Source: three-view drawing plus pictorial views. Frame: mm from the lowest corner of the part. A direction names the side the tool comes from. Give positions to 0.01 mm unless a question says otherwise; leave off trailing zeros. Loops run counter-clockwise (first coordinate to the right, second up) from the corner with the lowest first, then second, coordinate; pieces in that order, holes last. Notation, with made-up numbers: M -30.75,-24 L -26.75,-24 A20 cw -26.75,-19 Z; hole C 89.25,22 d2. An arc over 180 degrees is marked long. Put each result on its own line as item: value. Start each with the question number.
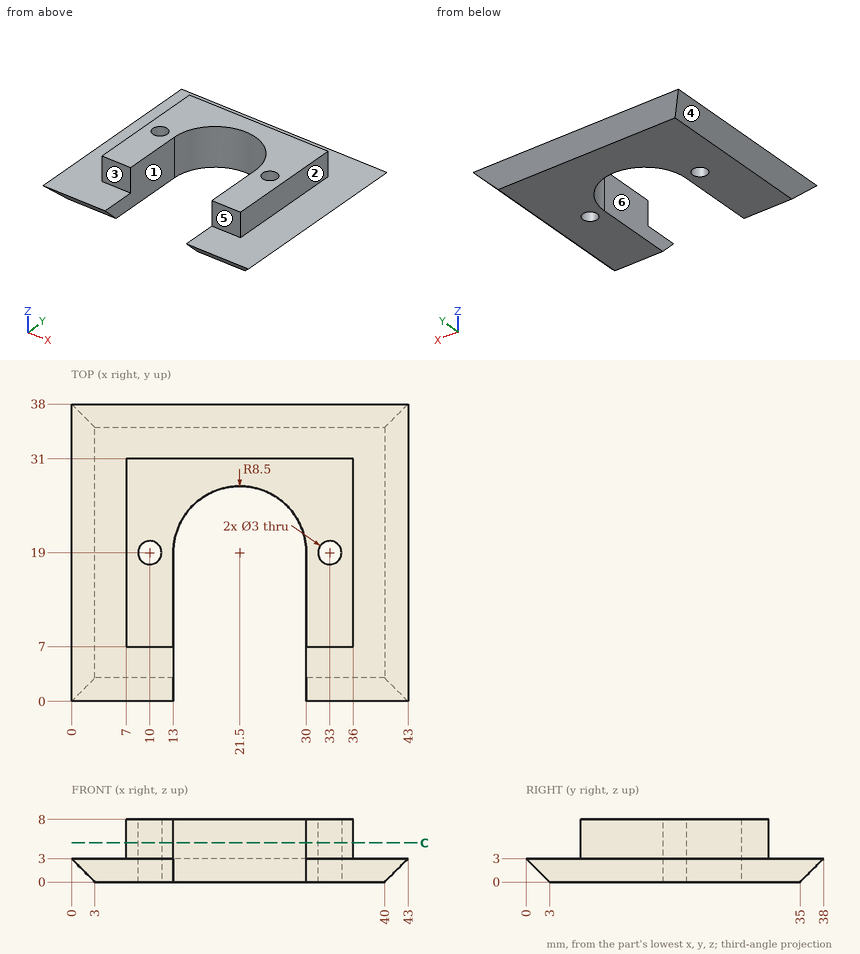
1. Section C-C, the plane z = 5. Output: boundary loops of the cut face in (x, y), plus the area to 3 significant figures.
2. Ray query, line 1 (Y direction, x = 33, z = 4); line 2 (X direction, y = 14.5, z = 7.5); line 3 (X direction, y = 18.5, z = 4.75). Return the intervals inside material, ascending.
3. Set-up query: the marked faces 1, 2 and 3. Return all of +Z, -Z, +X, -X, +Y, -Y with unobstructed straight access to the full face (end or side cutting, diameter ignored); none if empty.
4. Pull-direction query (X, two-part tool) for the marked faces 4, 5 and 6; classes: released by +X, released by -X, zero draft, split by the parting line, or undercut.
5. Contact query for flat-ended pins moving along their axis: pin 1 (3 mm diameter, centred on x = 31, z = 6, fed in from -Y); pin 2 (2.5 mm diameter, centred on y = 5.5, z = 2.5, fed in from -X); pin 3 (1.5 mm diameter, centred on y = 17.5, z = 6, fed in from +X); pin 4 (2.5 mm diameter, centred on x = 10, y = 19, fed in from -Z). Output: stop coordinate, or through.
Results found:
1. outline: M 7,7 L 13,7 L 13,19 A8.5 cw 30,19 L 30,7 L 36,7 L 36,31 L 7,31 Z; hole C 10,19 d3; hole C 33,19 d3
1. area: 364 mm²
2. line 1: 7 to 17.5, 20.5 to 31
2. line 2: 7 to 13, 30 to 36
2. line 3: 7 to 8.59, 11.41 to 13, 30 to 31.59, 34.41 to 36
3. face 1: +Z, -Z, -Y
3. face 2: +Z, +X, +Y, -Y
3. face 3: +Z, +X, -X, -Y
4. face 4: released by -X
4. face 5: zero draft
4. face 6: undercut
5. pin 1: y = 7
5. pin 2: x = 0
5. pin 3: x = 36
5. pin 4: through
